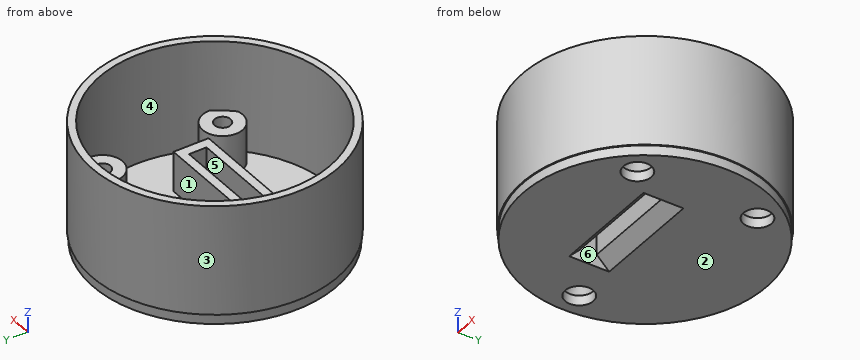
```python
from build123d import *

# Parameters (mm, degrees)
BOX002_W               = 22
BOX002_H               = 10
BOX002_DEPTH           = 10
BOX002_PLACEMENT_ANGLE = 45
CYLINDER010_R          = 1.6
CYLINDER010_DEPTH      = 10
CYLINDER009_R          = 2.8
CYLINDER009_DEPTH      = 2
CYLINDER008_R          = 4
CYLINDER008_DEPTH      = 8
CYLINDER007_R          = 1.6
CYLINDER007_DEPTH      = 10
CYLINDER006_R          = 2.8
CYLINDER006_DEPTH      = 2
CYLINDER005_R          = 4
CYLINDER005_DEPTH      = 8
CYLINDER004_R          = 1.6
CYLINDER004_DEPTH      = 10
CYLINDER003_R          = 2.8
CYLINDER003_DEPTH      = 2
CYLINDER001_R          = 4
CYLINDER001_DEPTH      = 8
BOX001_W               = 22
BOX001_H               = 3.5
BOX001_DEPTH           = 15
BOX_W                  = 26
BOX_H                  = 7
BOX_DEPTH              = 8
TUBE_R                 = 24.5
TUBE_R_2               = 23
TUBE_DEPTH             = 22
CYLINDER_R             = 24.3
CYLINDER_DEPTH         = 2


with BuildPart() as box002:
    # Box002 → Box002 (new body)
    with BuildSketch(Plane.XY):
        with Locations((11, 5)):
            Rectangle(BOX002_W, BOX002_H)
    extrude(amount=BOX002_DEPTH)


with BuildPart() as box002_1:
    # Box002 placement: moved
    add(box002.part.moved(Location((-11, -3.75, -10.15))).rotate(Axis((-11, -3.75, -10.15), (1, 0, 0)), BOX002_PLACEMENT_ANGLE))


with BuildPart() as cylinder010:
    # Cylinder010 → Cylinder010 (new body)
    with BuildSketch(Plane(origin=(15.5, -12, 0), x_dir=(1, 0, 0), z_dir=(0, 0, 1))):
        Circle(CYLINDER010_R)
    extrude(amount=CYLINDER010_DEPTH)


with BuildPart() as cone002:
    # Cone002 → Cone002 (revolve)
    with BuildSketch(Plane(origin=(15.5, -12, 2), x_dir=(1, 0, 0), z_dir=(0, -1, 0))):
        Polygon((0, 0), (2.8, 0), (0, 5.6), align=None)
    revolve(axis=Axis((15.5, -12, 2), (0, 0, 1)))


with BuildPart() as cylinder009:
    # Cylinder009 → Cylinder009 (new body)
    with BuildSketch(Plane(origin=(15.5, -12, 0), x_dir=(1, 0, 0), z_dir=(0, 0, 1))):
        Circle(CYLINDER009_R)
    extrude(amount=CYLINDER009_DEPTH)


with BuildPart() as cylinder008:
    # Cylinder008 → Cylinder008 (new body)
    with BuildSketch(Plane(origin=(15.5, -12, 2), x_dir=(1, 0, 0), z_dir=(0, 0, 1))):
        Circle(CYLINDER008_R)
    extrude(amount=CYLINDER008_DEPTH)


with BuildPart() as cylinder007:
    # Cylinder007 → Cylinder007 (new body)
    with BuildSketch(Plane(origin=(15.5, 12, 0), x_dir=(1, 0, 0), z_dir=(0, 0, 1))):
        Circle(CYLINDER007_R)
    extrude(amount=CYLINDER007_DEPTH)


with BuildPart() as cone001:
    # Cone001 → Cone001 (revolve)
    with BuildSketch(Plane(origin=(15.5, 12, 2), x_dir=(1, 0, 0), z_dir=(0, -1, 0))):
        Polygon((0, 0), (2.8, 0), (0, 5.6), align=None)
    revolve(axis=Axis((15.5, 12, 2), (0, 0, 1)))


with BuildPart() as cylinder006:
    # Cylinder006 → Cylinder006 (new body)
    with BuildSketch(Plane(origin=(15.5, 12, 0), x_dir=(1, 0, 0), z_dir=(0, 0, 1))):
        Circle(CYLINDER006_R)
    extrude(amount=CYLINDER006_DEPTH)


with BuildPart() as cylinder005:
    # Cylinder005 → Cylinder005 (new body)
    with BuildSketch(Plane(origin=(15.5, 12, 2), x_dir=(1, 0, 0), z_dir=(0, 0, 1))):
        Circle(CYLINDER005_R)
    extrude(amount=CYLINDER005_DEPTH)


with BuildPart() as cylinder004:
    # Cylinder004 → Cylinder004 (new body)
    with BuildSketch(Plane(origin=(-19.5, 0, 0), x_dir=(1, 0, 0), z_dir=(0, 0, 1))):
        Circle(CYLINDER004_R)
    extrude(amount=CYLINDER004_DEPTH)


with BuildPart() as cone:
    # Cone → Cone (revolve)
    with BuildSketch(Plane(origin=(-19.5, 0, 2), x_dir=(1, 0, 0), z_dir=(0, -1, 0))):
        Polygon((0, 0), (2.8, 0), (0, 5.6), align=None)
    revolve(axis=Axis((-19.5, 0, 2), (0, 0, 1)))


with BuildPart() as cylinder003:
    # Cylinder003 → Cylinder003 (new body)
    with BuildSketch(Plane(origin=(-19.5, 0, 0), x_dir=(1, 0, 0), z_dir=(0, 0, 1))):
        Circle(CYLINDER003_R)
    extrude(amount=CYLINDER003_DEPTH)


with BuildPart() as cylinder001:
    # Cylinder001 → Cylinder001 (new body)
    with BuildSketch(Plane(origin=(-19.5, 0, 2), x_dir=(1, 0, 0), z_dir=(0, 0, 1))):
        Circle(CYLINDER001_R)
    extrude(amount=CYLINDER001_DEPTH)


with BuildPart() as box001:
    # Box001 → Box001 (new body)
    with BuildSketch(Plane(origin=(-11, -5.75, -1), x_dir=(1, 0, 0), z_dir=(0, 0, 1))):
        with Locations((11, 1.75)):
            Rectangle(BOX001_W, BOX001_H)
    extrude(amount=BOX001_DEPTH)


with BuildPart() as box:
    # Box → Box (new body)
    with BuildSketch(Plane(origin=(-13, -7.5, 2), x_dir=(1, 0, 0), z_dir=(0, 0, 1))):
        with Locations((13, 3.5)):
            Rectangle(BOX_W, BOX_H)
    extrude(amount=BOX_DEPTH)


with BuildPart() as tube:
    # Tube → Tube (new body)
    with BuildSketch(Plane.XY.offset(2)):
        Circle(TUBE_R)
        Circle(TUBE_R_2, mode=Mode.SUBTRACT)
    extrude(amount=TUBE_DEPTH)


with BuildPart() as cut010:
    # Cylinder → Cylinder (new body)
    with BuildSketch(Plane.XY):
        Circle(CYLINDER_R)
    extrude(amount=CYLINDER_DEPTH)

    # Fusion: union Tube
    add(tube.part)

    # Fusion001: union Box
    add(box.part)

    # Cut: cut Box001
    add(box001.part, mode=Mode.SUBTRACT)

    # Fusion002: union Cylinder001
    add(cylinder001.part)

    # Cut001: cut Cylinder003
    add(cylinder003.part, mode=Mode.SUBTRACT)

    # Cut002: cut Cone
    add(cone.part, mode=Mode.SUBTRACT)

    # Cut003: cut Cylinder004
    add(cylinder004.part, mode=Mode.SUBTRACT)

    # Fusion003: union Cylinder005
    add(cylinder005.part)

    # Cut004: cut Cylinder006
    add(cylinder006.part, mode=Mode.SUBTRACT)

    # Cut005: cut Cone001
    add(cone001.part, mode=Mode.SUBTRACT)

    # Cut006: cut Cylinder007
    add(cylinder007.part, mode=Mode.SUBTRACT)

    # Fusion004: union Cylinder008
    add(cylinder008.part)

    # Cut007: cut Cylinder009
    add(cylinder009.part, mode=Mode.SUBTRACT)

    # Cut008: cut Cone002
    add(cone002.part, mode=Mode.SUBTRACT)

    # Cut009: cut Cylinder010
    add(cylinder010.part, mode=Mode.SUBTRACT)

    # Cut010: cut Box002
    add(box002_1.part, mode=Mode.SUBTRACT)


solid = cut010.part
```
Verification items for the finished model (mm, model axes). Face numbers are marked on the shaded views. A direction names the side the tool comes from. Coordinates: 2 decimals unless noted, no trailing zeros. Write each loop counter-clockwise with the first axis right and the second up, starting at its lowest first coordinate (ties: lowest second). Pieces come first, ordered by that corner, then holes. Notation, with made-up numbers: (52, -23) - (66, -23) arc R38 ccw to (66, 16) - close; hole circle Ø10 at (-11, 72). An arc over 180 degrees is marked (long way). Write item = value, one per line.
Q1. Mould release check, pull along X, two halves, no side actions. Record for the marked faces 1, 2 and 3: released by +X, released by -X, zero draft, split by the parting line, or undercut.
Answer:
face_1 = undercut
face_2 = zero draft
face_3 = split by the parting line
Q2. Access from +Z, -Z, +X, -X, +Y, -Y to the whole of each face (thin tool, end or side, straight path). Record for the marked faces 4, 5 and 6.
Answer:
face_4 = +Z
face_5 = +Z, -Z
face_6 = -Z
Q3. Cross-section at B-B (z = 15.25). Enter the section's corners in (x, y).
Answer:
outline = circle Ø49 at (0, 0); hole circle Ø46 at (0, 0)
Q4. Material ranges on L1, parallel to Y at x = -19.5, z = 7.55; L2, parallel to X at y = -10, z = 9; L3, parallel to Y at x = 15.5, z = 0.85, recorded low to high. Write a range as from..to.
Answer:
L1 = -14.83..-12.2, -4..-1.6, 1.6..4, 12.2..14.83
L2 = -22.37..-20.71, 12.04..18.96, 20.71..22.37
L3 = -18.71..-14.8, -9.2..9.2, 14.8..18.71
Q5. Cross-section at A-A (x = -5). Enter the section's corners in (y, z), plus the area to 3 significant figures.
Answer:
outline = (-23.98, 2) - (-23.78, 2) - (-23.78, 0) - (-7.74, 0) - (-5.75, 1.99) - (-5.75, 10) - (-7.5, 10) - (-7.5, 2) - (-22.45, 2) - (-22.45, 24) - (-23.98, 24) - close; (-2.25, 2.49) - (0.24, 0) - (23.78, 0) - (23.78, 2) - (23.98, 2) - (23.98, 24) - (22.45, 24) - (22.45, 2) - (-0.5, 2) - (-0.5, 10) - (-2.25, 10) - close
area = 179 mm²
Q6. Go/stop test with flat-tipped pins: pin 1 Ø3 at (x, y) = (15.5, -12) entering from +Z; pin 2 Ø4 at (y, z) = (-7.5, 21) entering from -X; pin 3 Ø9 at (x, y) = (15, -10) entering from +Z; pin 4 Ø2 at (x, z) = (-6, 2.5) entering from -Y. Record where each tip stops, or that it passes through.
Answer:
pin_1 = through
pin_2 = -23.87
pin_3 = 10
pin_4 = -23.98
